Read the model definition and answer for the solid it produces. Units are mm, in the model's axes. Face numbers are marked on the shaded views. A direction names the side the tool comes from. Give positions to 0.01 mm unless a question says otherwise; leave off trailing zeros. Order: outer loops, then holes, each group sorted by start corner. A loop starts at its lowest first (then second) coordinate and runs counter-clockwise, first axis right, second up. Notation, with made-up numbers: (-1.75, 84.25) -> (33.25, 84.25) arc R9 cw to (33.25, 95.25) -> close; hole circle Ø9 at (46, 23). An arc over 180 degrees is marked (long way). One line per item, written item: value. Start each with the question number.
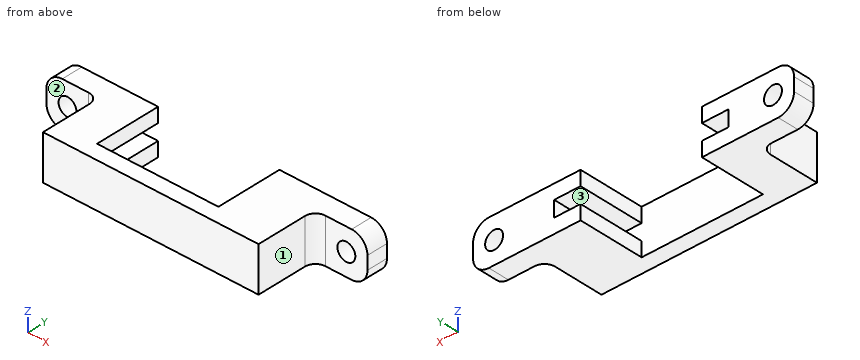
from build123d import *

# Parameters (mm, degrees)
SKETCH1_W           = 60.85
SKETCH1_H           = 8.5
BOSS_EXTRUDE1_DEPTH = 15.5
SKETCH4_R           = 1.7
CUT_EXTRUDE3_DEPTH  = 35.409201168
SKETCH2_W           = 5
SKETCH2_H           = 3
CUT_EXTRUDE1_DEPTH  = 12.5
SKETCH3_W           = 10
SKETCH3_H           = 8.5
CUT_EXTRUDE2_DEPTH  = 11.5
FILLET1_R           = 2
FILLET2_R           = 3


with BuildPart() as part:
    # Sketch1 → Boss-Extrude1 (new body)
    with BuildSketch(Plane(origin=(0, 0, 0), x_dir=(1, 0, 0), z_dir=(0, 1, 0))):
        Rectangle(SKETCH1_W, SKETCH1_H)
    extrude(amount=BOSS_EXTRUDE1_DEPTH)

    # Sketch4 → Cut-Extrude3 (cut, through all)
    with BuildSketch(Plane(origin=(0, 15.5, 0), x_dir=(1, 0, 0), z_dir=(0, 1, 0))):
        with Locations(Location((-26.425, 0, 0), (0, 0, 270))):
            Circle(SKETCH4_R)
        with Locations(Location((26.425, 0, 0), (0, 0, 90))):
            Circle(SKETCH4_R)
    extrude(amount=-CUT_EXTRUDE3_DEPTH, mode=Mode.SUBTRACT)

    # Sketch2 → Cut-Extrude1 (cut)
    with BuildSketch(Plane(origin=(0, 15.5, 0), x_dir=(1, 0, 0), z_dir=(0, 1, 0))):
        Polygon((-12.96, -1.5), (-12.96, -4.25), (10.04, -4.25), (10.04, -1.5), (10.04, 1.5), (10.04, 4.25), (-12.96, 4.25), (-12.96, 1.5), align=None)
        with Locations((-15.46, 0)):
            Rectangle(SKETCH2_W, SKETCH2_H)
        with Locations((12.54, 0)):
            Rectangle(SKETCH2_W, SKETCH2_H)
    extrude(amount=-CUT_EXTRUDE1_DEPTH, mode=Mode.SUBTRACT)

    # Sketch3 → Cut-Extrude2 (cut)
    with BuildSketch(Plane.XZ):
        with Locations((-25.425, 0)):
            Rectangle(SKETCH3_W, SKETCH3_H)
        with Locations((25.425, 0)):
            Rectangle(SKETCH3_W, SKETCH3_H)
    extrude(amount=-CUT_EXTRUDE2_DEPTH, mode=Mode.SUBTRACT)

    # Fillet1
    fillet1_edges = [part.edges().sort_by_distance(p)[0] for p in [
        (-20.425, 11.5, 0),
        (20.425, 11.5, 0),
    ]]
    fillet(fillet1_edges, radius=FILLET1_R)

    # Fillet2
    fillet2_edges = [part.edges().sort_by_distance(p)[0] for p in [
        (30.425, 13.5, 4.25),
        (-30.425, 13.5, 4.25),
        (-30.425, 13.5, -4.25),
        (30.425, 13.5, -4.25),
    ]]
    fillet(fillet2_edges, radius=FILLET2_R)


solid = part.part
Item 1: Find the intervals of material crossed by line 1 (X direction, y = 14.2, z = 0) (3 decimals); line 2 (Z direction, x = -15.5, y = 6.5); line 3 (X direction, y = 13, z = 0.75) (3 decimals), in increasing order. Write a range as from..to.
Item 2: A tool of negligible diameter and unlimited length cuts with its end or side. For the marked faces 1, 2 and 3, from which of +Z, -Z, +X, -X, +Y, -Y can it reach the whole face along a straight path? Write none if from no direction.
Item 3: Find section C-C on x = -3. Write down the section's boundary in (y, z), then the cut area to 3 significant figures.
Item 4: Flat-ended cylindrical pins translate along their axes: pin 1 (4 mm diameter, centred on x = 26.425, z = 0, fed in from +Y); pin 2 (3 mm diameter, centred on x = -24.5, y = 9, fed in from -Z); pin 3 (1.4 mm diameter, centred on y = 12, z = 3.5, fed in from -X); pin 4 (4 mm diameter, centred on y = 5.5, z = -2, fed in from -X) (3 decimals). Find the tip coordinate at first contact, or state that the pin passes through.
Item 5: Find section A-A on z = 0. Write down the section's boundary in (x, y) (3 decimals), then the cut area to 3 significant figures.
Item 6: Find section D-D on z = 3.5. Write down the section's boundary in (x, y) (3 decimals).
Item 7: Find section B-B on y = 13.75. Write down the section's boundary in (x, z) (3 decimals).
Checks:
1. line 1: -30.425..-28.125, -24.725..-17.96, 15.04..24.725, 28.125..30.425
1. line 2: -4.25..-1.5, 1.5..4.25
1. line 3: -30.425..-27.951, -24.899..-17.96, 15.04..24.899, 27.951..30.425
2. face 1: +Z, -Z, +X, -Y
2. face 2: +Z, -Z, -X, -Y
2. face 3: +Y
3. outline: (0, -4.25) -> (3, -4.25) -> (3, 4.25) -> (0, 4.25) -> close
3. area: 25.5 mm2
4. pin 1: y = 15.5
4. pin 2: through
4. pin 3: x = -29.99
4. pin 4: x = -20.425
5. outline: (-30.425, 11.5) -> (-28.125, 11.5) -> (-28.125, 15.5) -> (-30.425, 15.5) -> close; (-24.725, 11.5) -> (-22.425, 11.5) arc R2 cw to (-20.425, 9.5) -> (-20.425, 0) -> (20.425, 0) -> (20.425, 9.5) arc R2 cw to (22.425, 11.5) -> (24.725, 11.5) -> (24.725, 15.5) -> (15.04, 15.5) -> (15.04, 3) -> (-17.96, 3) -> (-17.96, 15.5) -> (-24.725, 15.5) -> close; (28.125, 11.5) -> (30.425, 11.5) -> (30.425, 15.5) -> (28.125, 15.5) -> close
5. area: 275 mm2
6. outline: (-29.409, 11.5) -> (-22.425, 11.5) arc R2 cw to (-20.425, 9.5) -> (-20.425, 0) -> (20.425, 0) -> (20.425, 9.5) arc R2 cw to (22.425, 11.5) -> (29.409, 11.5) -> (29.409, 15.5) -> (10.04, 15.5) -> (10.04, 3) -> (-12.96, 3) -> (-12.96, 15.5) -> (-29.409, 15.5) -> close
7. outline: (-30.425, -1.25) arc R3 ccw to (-27.425, -4.25) -> (-12.96, -4.25) -> (-12.96, -1.5) -> (-17.96, -1.5) -> (-17.96, 1.5) -> (-12.96, 1.5) -> (-12.96, 4.25) -> (-27.425, 4.25) arc R3 ccw to (-30.425, 1.25) -> close; (10.04, -4.25) -> (27.425, -4.25) arc R3 ccw to (30.425, -1.25) -> (30.425, 1.25) arc R3 ccw to (27.425, 4.25) -> (10.04, 4.25) -> (10.04, 1.5) -> (15.04, 1.5) -> (15.04, -1.5) -> (10.04, -1.5) -> close; hole circle Ø3.4 at (-26.425, 0); hole circle Ø3.4 at (26.425, 0)
